from build123d import *

# Parameters (mm, degrees)
SKETCH1_R           = 1.5
BOSS_EXTRUDE1_DEPTH = 2.35
BOSS_EXTRUDE2_START = -1
SKETCH2_R           = 1.5
SKETCH2_R_2         = 1.4
BOSS_EXTRUDE2_DEPTH = 1
CUT_EXTRUDE1_START  = -0.01
SKETCH3_R           = 1.5
SKETCH3_R_2         = 1.4
CUT_EXTRUDE1_DEPTH  = 0.01


with BuildPart() as part:
    # Sketch1 → Boss-Extrude1 (new body)
    with BuildSketch(Plane.XY):
        Polygon((2.085613633, -2.394483056), (3.116489972, 0.608952861), (1.030876339, 3.003435917), (-2.085613633, 2.394483056), (-3.116489972, -0.608952861), (-1.030876339, -3.003435917), align=None)
        Circle(SKETCH1_R, mode=Mode.SUBTRACT)
    extrude(amount=BOSS_EXTRUDE1_DEPTH)

    # Sketch2 → Boss-Extrude2 (add)
    with BuildSketch(Plane.XY.offset(2.35).offset(BOSS_EXTRUDE2_START)):
        Circle(SKETCH2_R)
        Circle(SKETCH2_R_2, mode=Mode.SUBTRACT)
    extrude(amount=BOSS_EXTRUDE2_DEPTH)

    # Sketch3 → Cut-Extrude1 (cut)
    with BuildSketch(Plane.XY.offset(2.35).offset(CUT_EXTRUDE1_START)):
        Circle(SKETCH3_R)
        Circle(SKETCH3_R_2, mode=Mode.SUBTRACT)
    extrude(amount=CUT_EXTRUDE1_DEPTH, mode=Mode.SUBTRACT)


solid = part.part
Model file for the job. Use its own axes, mm. A direction names the side the tool comes from. Give positions to 0.01 mm unless a question says otherwise; leave off trailing zeros. Loops run counter-clockwise (first coordinate to the right, second up) from the corner with the lowest first, then second, coordinate; pieces in that order, holes last.
1) Tool access for faces 4 (the cylindrical face through (-1.5, 0.07, 0.67)), 5 (the flat face through (-1.4, 1.4, 2.35)): list every direction of +Z, -Z, +X, -X, +Y, -Y with a clear straight run to the whole face (end or side of a thin tool).
2) Saw through at A-A (z = 1). Write the cut outline in (x, y), plus the area to 3 significant figures.
3) Saw through at D-D (z = 2.2). Write the cut outline in (x, y), plus the area to 3 significant figures.
4) Wall check: line 1 (Y direction, x = 0, z = 0.7); line 2 (Y direction, x = 1, z = 0.85); line 3 (X direction, y = -0.75, z = 2.25). Give the ranges that are in metal, low to high.
5) Flat gauge pins, fed straight in: pin 1 Ø1.7 at (x, y) = (0, 0) entering from +Z; pin 2 Ø1 at (x, z) = (-2.5, 1) entering from +Y. Where does each tip first touch, or does it go through?
6) Pull direction X, two halves, no side cores. Call faces 1 (the flat face through (-2.6, 0.9, 1.2)), 2 (the cylindrical face through (-1.4, 0.06, 1.84)), 3 (the flat face through (2.09, 1.79, 1.16)): +X half, -X half, draft (parallel to the pull), parting line (faces both ways), or undercut.
Answer block:
1. face 4: -Z
1. face 5: +Z, +X, -X, +Y, -Y
2. outline: (-3.12, -0.61) - (-1.03, -3) - (2.09, -2.39) - (3.12, 0.61) - (1.03, 3) - (-2.09, 2.39) - close; hole circle Ø3 at (0, 0)
2. area: 19.1 mm2
3. outline: (-3.12, -0.61) - (-1.03, -3) - (2.09, -2.39) - (3.12, 0.61) - (1.03, 3) - (-2.09, 2.39) - close; hole circle Ø2.8 at (0, 0)
3. area: 20.0 mm2
4. line 1: y = -2.8 to -1.5, 1.5 to 2.8
4. line 2: y = -2.61 to -1.12, 1.12 to 3
4. line 3: x = -2.99 to -1.18, 1.18 to 2.65
5. pin 1: passes through
5. pin 2: stops at y = 2.41
6. face 1: -X half
6. face 2: undercut
6. face 3: +X half
